Source: CAD feature listing. Evaluate the final solid. Frame: model axes, mm. Give positions to 0.01 mm unless a question says otherwise; leave off trailing zeros. Write each loop counter-clockwise with the first axis right and the second up, starting at its lowest first coordinate (ties: lowest second). Pieces come first, ordered by that corner, then holes. Notation, with made-up numbers: (-2.5, -31.5) - (17.5, -31.5) arc R24 ccw to (17.5, -17.5) - close; hole circle Ø5 at (56.25, 6). An arc over 180 degrees is marked (long way). One line per question, with ' | ' between items. Start each with the question number.
(1) Pin query (flat end, axial travel): pin 1 (3 mm diameter, centred on x = 23.5, y = 28.5, fed in from +Z). Return the tip coordinate at first contact, or that it passes through.
(2) Section C-C, the plane z = 7.5. Return loops of the section in (x, y), plus the area to 3 significant figures.
(3) Draft query along Y for faces 1 (the cylindrical face through (-0.477, 31.057, 1.247)), 2 (the flat face through (-0.477, 38.78, 1.282)), 3 (the flat face through (-34.064, 34, 2)). Return one class per face: +Y half, -Y half, draft (parallel to the pull), parting line (faces both ways), or undercut.
(4) Section D-D, the plane y = 37.25. Return loops of the section in (x, z).
(5) Ray query, line 1 (Z direction, x = 13, y = 33.5); line 2 (Y direction, x = -4.5, z = 10); line 3 (Z direction, x = -29, y = 36.75). Return the intervals inside material, ascending. Write a range as [from, to].
(6) Section A-A, the plane z = 5. Return loops of the section in (x, y), plus the area to 3 significant figures.
```python
from build123d import *

# Parameters (mm, degrees)
BOSS_EXTRUDE1_START = -34.064
SKETCH2_R           = 2.921
BOSS_EXTRUDE1_DEPTH = 68.128


with BuildPart() as part:
    # Sketch2 → Boss-Extrude1 (new body)
    with BuildSketch(Plane(origin=(0, 0, 0), x_dir=(0, 0, -1), z_dir=(1, 0, 0)).offset(BOSS_EXTRUDE1_START)):
        with BuildLine():
            Line((-1.82176, 39.714214029), (-3.950444551, 39.714214029))
            ThreePointArc((-3.950444551, 39.714214029), (-5.410944551, 38.323564029), (-6.871444551, 39.714214029))
            Line((-6.871444551, 39.714214029), (-9.000129101, 39.714214029))
            Line((-9.000129101, 39.714214029), (-10.064471377, 37.870719131))
            ThreePointArc((-10.064471377, 37.870719131), (-9.590383149, 35.910564029), (-11.524971377, 35.341058926))
            Line((-11.524971377, 35.341058926), (-12.589313652, 33.497564029))
            Line((-12.589313652, 33.497564029), (-11.524971377, 31.654069131))
            ThreePointArc((-11.524971377, 31.654069131), (-9.590383149, 31.084564029), (-10.064471377, 29.124408926))
            Line((-10.064471377, 29.124408926), (-9.000129101, 27.280914029))
            Line((-9.000129101, 27.280914029), (-6.871444551, 27.280914029))
            ThreePointArc((-6.871444551, 27.280914029), (-5.410944551, 28.671564029), (-3.950444551, 27.280914029))
            Line((-3.950444551, 27.280914029), (-1.82176, 27.280914029))
            Line((-1.82176, 27.280914029), (-0.757417724, 29.124408926))
            ThreePointArc((-0.757417724, 29.124408926), (-1.231505952, 31.084564029), (0.703082276, 31.654069131))
            Line((0.703082276, 31.654069131), (1.767424551, 33.497564029))
            Line((1.767424551, 33.497564029), (0.703082276, 35.341058926))
            ThreePointArc((0.703082276, 35.341058926), (-1.231505952, 35.910564029), (-0.757417724, 37.870719131))
            Line((-0.757417724, 37.870719131), (-1.82176, 39.714214029))
        make_face()
        with Locations((-5.410944551, 33.497564029)):
            Circle(SKETCH2_R, mode=Mode.SUBTRACT)
    extrude(amount=BOSS_EXTRUDE1_DEPTH)


solid = part.part
```
Check sheet entries:
1) pin 1: z = 10.06
2) outline: (-34.06, 27.28) - (34.06, 27.28) - (34.06, 31.46) - (-34.06, 31.46) - close; (-34.06, 35.54) - (34.06, 35.54) - (34.06, 39.71) - (-34.06, 39.71) - close | area: 569 mm²
3) face 1: undercut | face 2: +Y half | face 3: draft
4) outline: (-34.06, 1.29) - (34.06, 1.29) - (34.06, 9.53) - (-34.06, 9.53) - close
5) line 1: [-1.77, 2.49], [8.33, 12.59] | line 2: [29.01, 29.17], [31.54, 35.46], [37.83, 37.98] | line 3: [1.42, 9.4]
6) outline: (-34.06, 28.61) - (34.06, 28.61) - (34.06, 30.61) - (-34.06, 30.61) - close; (-34.06, 36.39) - (34.06, 36.39) - (34.06, 38.38) - (-34.06, 38.38) - close | area: 272 mm²
